Verification items for the finished model (mm, model axes). Face numbers are marked on the shaded views. Give positions to 0.01 mm unless a question says otherwise; leave off trailing zeros. Loops run counter-clockwise (first coordinate to the right, second up) from the corner with the lowest first, then second, coordinate; pieces in that order, holes last. Notation, with made-up numbers: (13.5, -31) - (28.5, -31) arc R20 cw to (28.5, -11) - close; hole circle Ø2 at (-10, 71.25). An arc over 180 degrees is marked (long way). One line per item, written item: value. Start each with the question number.
1. Sectioned sample at C-C (z = -0.9). Count the separate pieces of the cut face and the enclosed holes in it, plus the area to 3 significant figures.
2. Sectioned sample at A-A (y = 0). Record the cut outline in (x, z).
3. Sectioned sample at D-D (x = 10). Record the cut outline in (y, z).
4. Scan lines: L1, parallel to Y at x = 44.5, z = -1.25; L2, parallel to X at y = 0.5, z = -0.7; L3, parallel to X at y = -50, z = -0.45 (3 decimals). Record each from-to range of solid material in increasing order. Write a range as [from, to].
5. Gauge pin test, flat ends, axial feed: pin 1 (0.8 mm diameter, centred on x = 5.5, z = -1, fed in from +Y); pin 2 (6 mm diameter, centred on x = 24, y = 21, fed in from -Z); pin 3 (0.8 mm diameter, centred on y = 8, z = -1, fed in from +X). Record the tip position at first contact, or that the pin passes through.
6. Mould release check, pull along Y, two halves, no side actions. Record for the marked faces 1 and 2: pulls with the +Y half, pulls with the -Y half, needs draft (parallel to the pull), parting line crosses it, or undercut.
from build123d import *

# Parameters (mm, degrees)
SKETCH_W      = 110
SKETCH_H      = 110
PAD_DEPTH     = 1.5
PAD001_DEPTH  = 1.5
SKETCH002_R   = 5
SKETCH002_R_2 = 1.5
PAD002_DEPTH  = 1.5


with BuildPart() as part:
    # Sketch → Pad (new body)
    with BuildSketch(Plane.XY):
        Rectangle(SKETCH_W, SKETCH_H)
    extrude(amount=PAD_DEPTH)

    # Sketch001 → Pad001 (join)
    with BuildSketch(Plane(origin=(0, 0, 0), x_dir=(1, 0, 0), z_dir=(0, 0, -1))):
        with BuildLine():
            Line((-49.8, 53.8), (49.8, 53.8))
            ThreePointArc((53.8, 49.8), (52.628427, 52.628427), (49.8, 53.8))
            Line((53.8, 49.8), (53.8, -49.8))
            ThreePointArc((49.8, -53.8), (52.628427, -52.628427), (53.8, -49.8))
            Line((49.8, -53.8), (-49.8, -53.8))
            ThreePointArc((-53.8, -49.8), (-52.628427, -52.628427), (-49.8, -53.8))
            Line((-53.8, -49.8), (-53.8, 49.8))
            ThreePointArc((-49.8, 53.8), (-52.628427, 52.628427), (-53.8, 49.8))
        make_face()
        with BuildLine():
            Line((-49.8, 52.8), (49.8, 52.8))
            ThreePointArc((52.8, 49.8), (51.92132, 51.92132), (49.8, 52.8))
            Line((52.8, 49.8), (52.8, -49.8))
            ThreePointArc((49.8, -52.8), (51.92132, -51.92132), (52.8, -49.8))
            Line((49.8, -52.8), (-49.8, -52.8))
            ThreePointArc((-52.8, -49.8), (-51.92132, -51.92132), (-49.8, -52.8))
            Line((-52.8, -49.8), (-52.8, 49.8))
            ThreePointArc((-49.8, 52.8), (-51.92132, 51.92132), (-52.8, 49.8))
        make_face(mode=Mode.SUBTRACT)
    extrude(amount=PAD001_DEPTH)

    # Sketch002 → Pad002 (join)
    with BuildSketch(Plane(origin=(0, 0, 0), x_dir=(1, 0, 0), z_dir=(0, 0, -1))):
        with Locations((-40.005, 40.005)):
            Circle(SKETCH002_R)
        with Locations((-40.005, 49.505)):
            Circle(SKETCH002_R_2)
        with Locations((-13.335, 40.005)):
            Circle(SKETCH002_R)
        with Locations((-13.335, 49.505)):
            Circle(SKETCH002_R_2)
        with Locations((13.335, 40.005)):
            Circle(SKETCH002_R)
        with Locations((13.335, 49.505)):
            Circle(SKETCH002_R_2)
        with Locations((40.005, 40.005)):
            Circle(SKETCH002_R)
        with Locations((40.005, 49.505)):
            Circle(SKETCH002_R_2)
        with Locations((-40.005, 13.335)):
            Circle(SKETCH002_R)
        with Locations((-40.005, 22.835)):
            Circle(SKETCH002_R_2)
        with Locations((-13.335, 13.335)):
            Circle(SKETCH002_R)
        with Locations((-13.335, 22.835)):
            Circle(SKETCH002_R_2)
        with Locations((13.335, 13.335)):
            Circle(SKETCH002_R)
        with Locations((13.335, 22.835)):
            Circle(SKETCH002_R_2)
        with Locations((40.005, 13.335)):
            Circle(SKETCH002_R)
        with Locations((40.005, 22.835)):
            Circle(SKETCH002_R_2)
        with Locations((-40.005, -13.335)):
            Circle(SKETCH002_R)
        with Locations((-40.005, -3.835)):
            Circle(SKETCH002_R_2)
        with Locations((-13.335, -13.335)):
            Circle(SKETCH002_R)
        with Locations((-13.335, -3.835)):
            Circle(SKETCH002_R_2)
        with Locations((13.335, -13.335)):
            Circle(SKETCH002_R)
        with Locations((13.335, -3.835)):
            Circle(SKETCH002_R_2)
        with Locations((40.005, -13.335)):
            Circle(SKETCH002_R)
        with Locations((40.005, -3.835)):
            Circle(SKETCH002_R_2)
        with Locations((-40.005, -40.005)):
            Circle(SKETCH002_R)
        with Locations((-40.005, -30.505)):
            Circle(SKETCH002_R_2)
        with Locations((-13.335, -40.005)):
            Circle(SKETCH002_R)
        with Locations((-13.335, -30.505)):
            Circle(SKETCH002_R_2)
        with Locations((13.335, -40.005)):
            Circle(SKETCH002_R)
        with Locations((13.335, -30.505)):
            Circle(SKETCH002_R_2)
        with Locations((40.005, -40.005)):
            Circle(SKETCH002_R)
        with Locations((40.005, -30.505)):
            Circle(SKETCH002_R_2)
    extrude(amount=PAD002_DEPTH)


solid = part.part
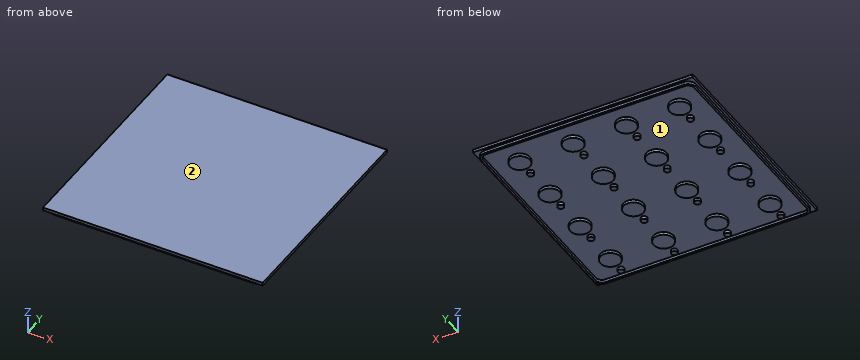
Results are:
1. separate pieces: 33
1. enclosed holes: 1
1. area: 1,790 mm^2
2. outline: (-55, 0) - (-53.8, 0) - (-53.8, -1.5) - (-52.8, -1.5) - (-52.8, 0) - (52.8, 0) - (52.8, -1.5) - (53.8, -1.5) - (53.8, 0) - (55, 0) - (55, 1.5) - (-55, 1.5) - close
3. outline: (-55, 0) - (-53.8, 0) - (-53.8, -1.5) - (-52.8, -1.5) - (-52.8, 0) - (-43.73, 0) - (-43.73, -1.5) - (-36.28, -1.5) - (-36.28, 0) - (-17.06, 0) - (-17.06, -1.5) - (-9.61, -1.5) - (-9.61, 0) - (9.61, 0) - (9.61, -1.5) - (17.06, -1.5) - (17.06, 0) - (36.28, 0) - (36.28, -1.5) - (43.73, -1.5) - (43.73, 0) - (52.8, 0) - (52.8, -1.5) - (53.8, -1.5) - (53.8, 0) - (55, 0) - (55, 1.5) - (-55, 1.5) - close
4. L1: y = [-53.8, -52.8], [-42.19, -37.82], [-15.52, -11.15], [11.15, 15.52], [37.82, 42.19], [52.8, 53.8]
4. L2: x = [-53.8, -52.8], [52.8, 53.8]
4. L3: x = [-53.795, -52.793], [-41.421, -38.589], [-14.751, -11.919], [11.919, 14.751], [38.589, 41.421], [52.793, 53.795]
5. pin 1: stops at y = 53.8
5. pin 2: stops at z = 0
5. pin 3: stops at x = 53.8
6. face 1: undercut
6. face 2: needs draft
